Autodesk Inventor part; units mm, degrees
ref_plane "YZ Plane" through (0, 0, 0) normal (1, 0, 0) x (0, 1, 0)
ref_plane "XZ Plane" through (0, 0, 0) normal (0, 1, 0) x (-1, 0, 0)
ref_plane "XY Plane" through (0, 0, 0) normal (0, 0, 1) x (1, 0, 0)
sketch "Sketch1" plane through (0, 0, 0) normal (0, 0, 1) x (1, 0, 0)
  line L0 (0, -7.5) -> (-6.4952, -3.75)
  line L1 (-6.4952, -3.75) -> (-6.4952, 3.75)
  line L2 (-6.4952, 3.75) -> (0, 7.5)
  line L3 (0, 7.5) -> (6.4952, 3.75)
  line L4 (6.4952, 3.75) -> (6.4952, -3.75)
  line L5 (6.4952, -3.75) -> (0, -7.5)
  line L6 (-2.5, -8.366) -> (-2.5, -24.8094)
  line L7 (-2.5, -24.8094) -> (-10, -24.8094)
  line L8 (-10, -24.8094) -> (-10, -27.8094)
  line L9 (10, -27.8094) -> (-10, -27.8094)
  line L10 (10, -24.8094) -> (10, -27.8094)
  line L11 (10, -24.8094) -> (2.5, -24.8094)
  line L12 (2.5, -24.8094) -> (2.5, -8.366)
  line L13 (2.5, -8.366) -> (8.4952, -4.9047)
  line L14 (8.4952, -4.9047) -> (33.544, -4.9047)
  arc A0 (33.544, -4.9047) -> (33.544, 4.9047) centre (37, 0) ccw
  line L15 (33.544, 4.9047) -> (8.4952, 4.9047)
  line L16 (8.4952, 4.9047) -> (0, 9.8094)
  line L17 (0, 9.8094) -> (-8.4952, 4.9047)
  line L18 (-8.4952, 4.9047) -> (-33.544, 4.9047)
  arc A1 (-33.544, 4.9047) -> (-33.544, -4.9047) centre (-37, 0) ccw
  line L19 (-33.544, -4.9047) -> (-8.4952, -4.9047)
  line L20 (-8.4952, -4.9047) -> (-2.5, -8.366)
  circle A2 centre (37, 0) radius 4.25
  circle A3 centre (-19.7476, 0) radius 2.5
  circle A4 centre (19.7476, 0) radius 2.5
  circle A5 centre (-37.0722, -0.0001) radius 4.25
  line L21 (6.4952, 3.75) -> (6.4952, -3.75)
  line L22 (0, 7.5) -> (6.4952, 3.75)
  line L23 (-6.4952, 3.75) -> (0, 7.5)
  line L24 (-6.4952, -3.75) -> (-6.4952, 3.75)
  line L25 (0, -7.5) -> (-6.4952, -3.75)
  line L26 (6.4952, -3.75) -> (0, -7.5)
  circle A6 centre (0, 0) radius 5
  line L27 (0, 9.8094) -> (8.4952, 4.9047)
  line L28 (8.4952, 4.9047) -> (8.4952, -4.9047)
  line L29 (8.4952, -4.9047) -> (0, -9.8094)
  line L30 (0, -9.8094) -> (-8.4952, -4.9047)
  line L31 (-8.4952, -4.9047) -> (-8.4952, 4.9047)
  line L32 (-8.4952, 4.9047) -> (0, 9.8094)
extrude "Extrusion1" add sketch "Sketch1" against normal blind 2 contours L0 L1 L2 L3 L4 L5 | L20 L31 L17 L16 L28 L13 L29 L30 | L19 A1 L18 L31 | L28 L15 A0 L14 | A2 | A3 | A4 | A5
extrude "Extrusion2" add sketch "Sketch1" along normal blind 10 contours L0 L1 L2 L3 L4 L5 | L20 L31 L17 L16 L28 L13 L29 L30 | L19 A1 L18 L31 | L28 L15 A0 L14 | A3 | A4
properties part number "chep_za_os"
Verification items for the finished model (mm, model axes). A direction names the side the tool comes from. Coordinates: 2 decimals unless noted, no trailing zeros. Order: outer loops, then holes, each group sorted by start corner. A loop starts at its lowest first (then second) coordinate and runs counter-clockwise, first axis right, second up. Notation, with made-up numbers: (-3.5, -29.75) -> (2.5, -29.75) arc R37 ccw to (2.5, 8.25) -> close; hole circle Ø5 at (86.5, -8.75). An arc over 180 degrees is marked (long way). Put each result on its own line as item: value. Start each with the question number.
1. Cross-section at B-B, the plane y = 1. Record the boundary of the cut face in (x, z), then the cut area to 3 significant figures.
2. Cross-section at C-C, the plane z = 9. Record the boundary of the cut face in (x, y), then the cut area to 3 significant figures.
3. Material ranges on L1, parallel to Y at x = 0, z = 2; L2, parallel to Y at x = 37, z = 6.5; L3, parallel to X at y = 0.75, z = 6.25, recorded low to high. Write a range as [from, to].
4. Cross-section at A-A, the plane x = 37. Record the boundary of the cut face in (y, z), then the cut area to 3 significant figures.
5. Access from +Z, -Z, +X, -X, +Y, -Y to the whole of each face (thin tool, end or side, straight path). Record for faces 4 (the cylindrical face through (-33.02, -1.28, 4.93)), 5 (the flat face through (21, -4.905, 4)), 6 (the flat face through (21, 4.905, 4)), 7 (the cylindrical face through (-43, 0, 4)).
6. Go/stop test with flat-tipped pins: pin 1 Ø6 at (x, z) = (24, 3.5) entering from -Y; pin 2 Ø3.5 at (x, z) = (25, 2.5) entering from +Y; pin 3 Ø1 at (y, z) = (7.5, -0.5) entering from -X. Record where each tip stops, or that it passes through.
7. Mould release check, pull along Y, two halves, no side actions. Record for faces 1 (the cylindrical face through (43, 0, 4)), 2 (the flat face through (-21, -4.905, 4)), 3 (the flat face through (-37, 0, 0)): released by +Y, released by -Y, zero draft, split by the parting line, or undercut.
8. Cross-section at D-D, the plane y = -7.25. Record the boundary of the cut face in (x, z).
Computed:
1. outline: (-42.92, -2) -> (-4.9, -2) -> (-4.9, 10) -> (-32.94, 10) -> (-32.94, 0) -> (-41.2, 0) -> (-41.2, 10) -> (-42.92, 10) -> close; (4.9, -2) -> (42.92, -2) -> (42.92, 10) -> (41.13, 10) -> (41.13, 0) -> (32.87, 0) -> (32.87, 10) -> (4.9, 10) -> close
1. area: 747 mm2
2. outline: (-33.54, -4.9) -> (-8.5, -4.9) -> (-2.5, -8.37) -> (0, -9.81) -> (2.5, -8.37) -> (8.5, -4.9) -> (33.54, -4.9) arc R6 ccw (long way) to (33.54, 4.9) -> (8.5, 4.9) -> (0, 9.81) -> (-8.5, 4.9) -> (-33.54, 4.9) arc R6 ccw (long way) to start; hole circle Ø8.5 at (-37.07, 0); hole circle Ø10 at (0, 0); hole circle Ø8.5 at (37, 0)
2. area: 741 mm2
3. L1: [-9.81, -5], [5, 9.81]
3. L2: [-6, -4.25], [4.25, 6]
3. L3: [-42.95, -41.26], [-32.89, -4.94], [4.94, 32.82], [41.18, 42.95]
4. outline: (-6, -2) -> (6, -2) -> (6, 10) -> (4.25, 10) -> (4.25, 0) -> (-4.25, 0) -> (-4.25, 10) -> (-6, 10) -> close
4. area: 59.0 mm2
5. face 4: +Z
5. face 5: +Z, -Z, -Y
5. face 6: +Z, -Z, +Y
5. face 7: +Z, -Z
6. pin 1: y = -4.9
6. pin 2: y = 4.9
6. pin 3: x = -4.87
7. face 1: split by the parting line
7. face 2: released by -Y
7. face 3: undercut
8. outline: (-4.43, -2) -> (4.43, -2) -> (4.43, 10) -> (-4.43, 10) -> close
